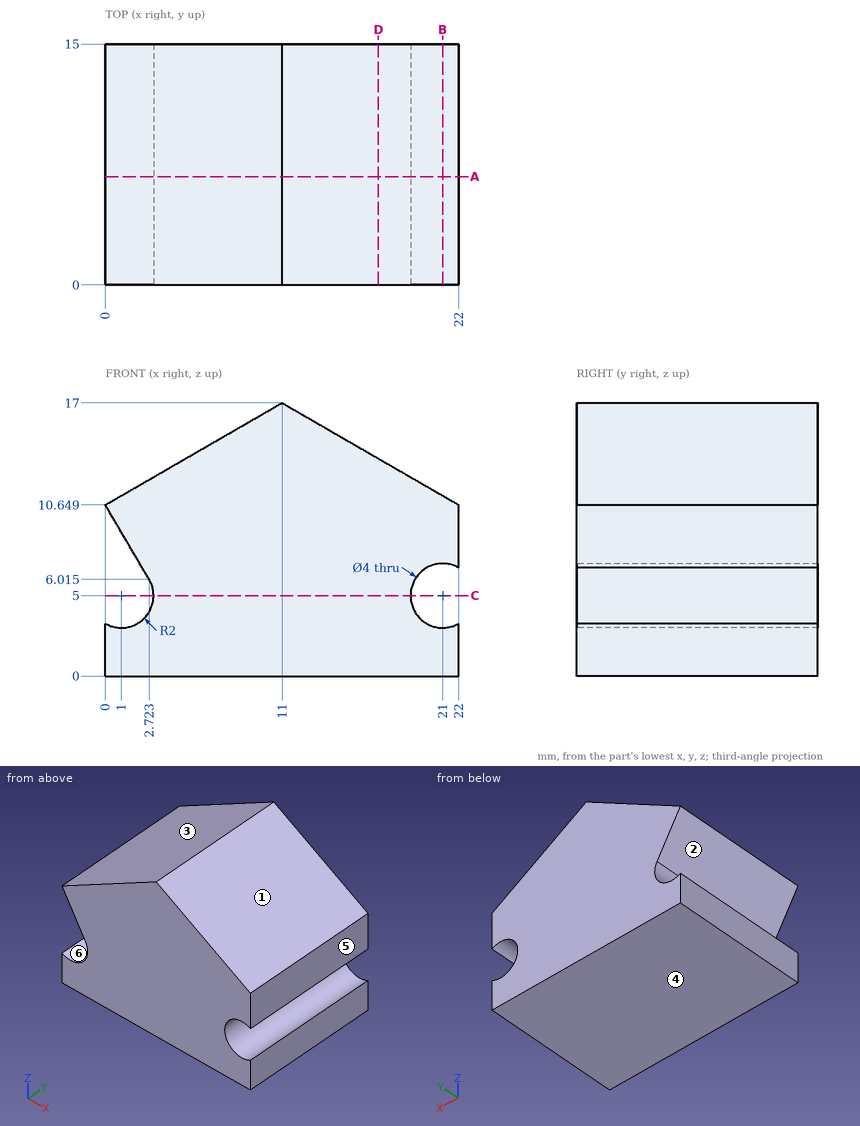
Verification items for this drawing (mm, ordinates from the low corner). A direction names the side the tool comes from. Round coordinates to 2 decimals unless told otherwise and drop trailing zeros. Loops run counter-clockwise (first coordinate to the right, second up) from the corner with the lowest first, then second, coordinate; pieces in that order, holes last. Notation, with made-up numbers: M -12,39 L 26,39 A24 ccw 26,61 Z; hole C -33,17 d10. An arc over 180 degrees is marked long. Answer as a JSON object with one key per item and string values.
1. Scan lines: line 1 (Z direction, x = 21, y = 11.25) (1 decimal); line 2 (X direction, y = 9.75, z = 10); line 3 (Z direction, x = 17.5, y = 3). Record each from-to range of solid material in increasing order.
Reply:
{"line 1": "z = 0 to 3, 7 to 11.2", "line 2": "x = 0.38 to 22", "line 3": "z = 0 to 13.25"}
2. Section check D-D (x = 17). Record the boundary of the cut face in (y, z).
Reply:
{"outline": "M 0,0 L 15,0 L 15,13.54 L 0,13.54 Z"}
3. Mould release check, pull along X, two halves, no side actions. Record for the marked faces 3, 4, 5 and 6: pulls with the +X half, pulls with the -X half, needs draft (parallel to the pull), parting line crosses it, or undercut.
Reply:
{"face 3": "pulls with the -X half", "face 4": "needs draft", "face 5": "pulls with the +X half", "face 6": "undercut"}
4. Section check B-B (x = 21). Record the boundary of the cut face in (y, z), plus the area to 3 significant figures.
Reply:
{"outline": "M 0,0 L 15,0 L 15,3 L 0,3 Z; M 0,7 L 15,7 L 15,11.23 L 0,11.23 Z", "area": "108 mm²"}
5. Access from +Z, -Z, +X, -X, +Y, -Y to the whole of each face (thin tool, end or side, straight path). Record for the marked faces 1 and 2.
Reply:
{"face 1": "+Z, +X, +Y, -Y", "face 2": "-X, +Y, -Y"}
6. Section check C-C (z = 5). Record the boundary of the cut face in (x, y).
Reply:
{"outline": "M 3,0 L 19,0 L 19,15 L 3,15 Z"}
7. Gauge pin test, flat ends, axial feed: P1, Ø2, axis at x = 4.5, z = 14.5, coming from the -Y side; P2, Ø4, axis at x = 4, y = 2.5, coming from the +Z side; P3, Ø3, axis at y = 11, z = 14.5, coming from the +X side. Record the tip position at first contact, or that the pin passes through.
Reply:
{"P1": "passes through", "P2": "stops at z = 14.11", "P3": "stops at x = 17.93"}
8. Section check A-A (y = 6.75). Record the boundary of the cut face in (x, z) (1 decimal).
Reply:
{"outline": "M 0,0 L 22,0 L 22,3.3 A2 cw long 22,6.7 L 22,10.6 L 11,17 L 0,10.6 L 2.7,6 A2 cw 0,3.3 Z"}
